Model file for the job. Use its own axes, mm. Face numbers are marked on the shaded views. A direction names the side the tool comes from. Coordinates: 2 decimals unless noted, no trailing zeros. Order: outer loops, then holes, each group sorted by start corner. A loop starts at its lowest first (then second) coordinate and runs counter-clockwise, first axis right, second up. Notation, with made-up numbers: (-0.5, 63.25) -> (51.5, 63.25) arc R29 cw to (51.5, 83.25) -> close; hole circle Ø2 at (71, 76.25). An arc over 180 degrees is marked (long way). Write item = value, one per line. Start each with the question number.
Q1. Flat gauge pins, fed straight in: pin 1 (1.5 mm diameter, centred on x = -58, z = 4.5, fed in from +Y); pin 2 (6 mm diameter, centred on x = -53.5, y = 10, fed in from +Z); pin 3 (4 mm diameter, centred on x = -58, y = 5, fed in from +Z). Where does each tip first touch, or does it go through?
Q2. 3-axis set-ups, long thin cutter, end or side, ignore diameter. For the marked faces 1 and 2: which of +Z, -Z, +X, -X, +Y, -Y reach the whole face in a straight line?
Q3. Wall check: line 1 (X direction, y = 3.25, z = -0.25); line 2 (Y direction, x = -48.5, z = 6.25); line 3 (X direction, y = 0.75, z = -4). Give the ranges that are in metal, low to high. Write a range as from..to.
Q4. Cut at A-A, the plane y = 8. List the corners of the cut face in (x, z).
Q5. Cut at B-B, the plane y = 3.25. List the corners of the cut face in (x, z), plus the area to 3 significant figures.
from build123d import *

# Parameters (mm, degrees)
SKETCH1_R           = 8.5
BOSS_EXTRUDE1_DEPTH = 6
FILLET2_R           = 1
SKETCH2_R           = 5
BOSS_EXTRUDE3_DEPTH = 6
BOSS_EXTRUDE3_TAPER = 2
FILLET4_R           = 1


with BuildPart() as part:
    # Sketch1 → Boss-Extrude1 (new body)
    with BuildSketch(Plane(origin=(0, 0, 0), x_dir=(1, 0, 0), z_dir=(0, 1, 0))):
        with Locations(Location((-51.120170416, 0, 0), (0, 0, 270))):
            Circle(SKETCH1_R)
    extrude(amount=BOSS_EXTRUDE1_DEPTH)

    # Fillet2
    fillet2_edges = [part.edges().sort_by_distance(p)[0] for p in [
        (-51.120170416, 6, -8.5),
    ]]
    fillet(fillet2_edges, radius=FILLET2_R)

    # Sketch2 → Boss-Extrude3 (add)
    with BuildSketch(Plane(origin=(0, 6, 0), x_dir=(1, 0, 0), z_dir=(0, 1, 0))):
        with Locations((-51.120170416, 0)):
            Circle(SKETCH2_R)
    extrude(amount=BOSS_EXTRUDE3_DEPTH, taper=BOSS_EXTRUDE3_TAPER)

    # Fillet4
    fillet4_edges = [part.edges().sort_by_distance(p)[0] for p in [
        (-55.9106458, 12, 0),
    ]]
    fillet(fillet4_edges, radius=FILLET4_R)


solid = part.part
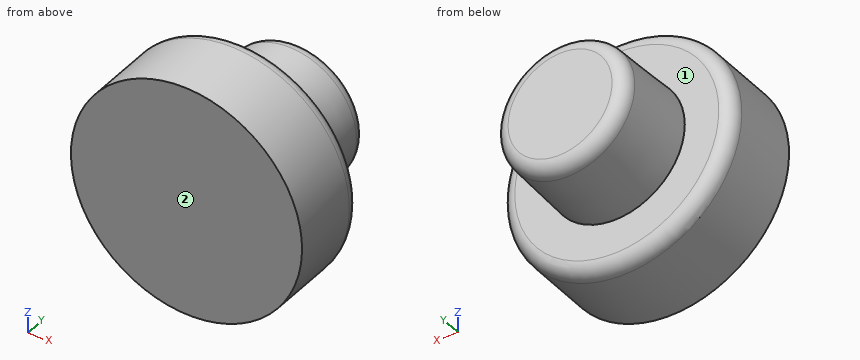
Here are the results:
q1.pin_1 = 6
q1.pin_2 = 4.93
q1.pin_3 = 6.96
q2.face_1 = +Y
q2.face_2 = +Z, -Z, +X, -X, -Y
q3.line_1 = -59.62..-42.62
q3.line_2 = 0..6
q3.line_3 = -58.62..-43.62
q4.outline = circle Ø9.86 at (-51.12, 0)
q5.outline = circle Ø17 at (-51.12, 0)
q5.area = 227 mm²
